```python
from build123d import *

# Parameters (mm, degrees)
SKETCH1_R           = 117.5
BOSS_EXTRUDE1_DEPTH = 5
SKETCH2_R           = 5.75
CUT_EXTRUDE1_DEPTH  = 167.245300685
CIRPATTERN1_COUNT   = 50
SKETCH3_R           = 6.25
CUT_EXTRUDE2_DEPTH  = 167.245300685
SKETCH4_R           = 2.25
CUT_EXTRUDE3_DEPTH  = 167.245300685
CIRPATTERN2_COUNT   = 4


with BuildPart() as part:
    # Sketch1 → Boss-Extrude1 (new body)
    with BuildSketch(Plane(origin=(0, 0, 0), x_dir=(1, 0, 0), z_dir=(0, 1, 0))):
        with Locations(Location((0, 0, 0), (0, 0, 270))):
            Circle(SKETCH1_R)
    extrude(amount=BOSS_EXTRUDE1_DEPTH)

    # Sketch2 → Cut-Extrude1 (cut, through all)
    with BuildSketch(Plane(origin=(0, 5, 0), x_dir=(1, 0, 0), z_dir=(0, 1, 0))):
        with Locations(Location((0, 107.5, 0), (0, 0, 270))):
            Circle(SKETCH2_R)
    cut_extrude1 = extrude(amount=-CUT_EXTRUDE1_DEPTH, mode=Mode.SUBTRACT)

    # CirPattern1: Cut-Extrude1 ×50 about axis
    cirpattern1_axis = Axis((0, 0, 0.258053464), (0, 1, 0))
    for i in range(1, CIRPATTERN1_COUNT):
        add(cut_extrude1.rotate(cirpattern1_axis, i * 360 / CIRPATTERN1_COUNT), mode=Mode.SUBTRACT)

    # Sketch3 → Cut-Extrude2 (cut, through all)
    with BuildSketch(Plane(origin=(0, 5, 0), x_dir=(1, 0, 0), z_dir=(0, 1, 0))):
        with Locations(Location((0, 0, 0), (0, 0, 270))):
            Circle(SKETCH3_R)
    extrude(amount=-CUT_EXTRUDE2_DEPTH, mode=Mode.SUBTRACT)

    # Sketch4 → Cut-Extrude3 (cut, through all)
    with BuildSketch(Plane(origin=(0, 5, 0), x_dir=(1, 0, 0), z_dir=(0, 1, 0))):
        with Locations(Location((19, 0, 0), (0, 0, 270))):
            Circle(SKETCH4_R)
    cut_extrude3 = extrude(amount=-CUT_EXTRUDE3_DEPTH, mode=Mode.SUBTRACT)

    # CirPattern2: Cut-Extrude3 ×4 about axis
    cirpattern2_axis = Axis((0, 0, 0), (0, 1, 0))
    for i in range(1, CIRPATTERN2_COUNT):
        add(cut_extrude3.rotate(cirpattern2_axis, i * 360 / CIRPATTERN2_COUNT), mode=Mode.SUBTRACT)


solid = part.part
```
Geometry check sheet. Reference: the model listing, model coordinates, mm. Coordinates: 2 decimals unless noted, no trailing zeros. Write each loop counter-clockwise with the first axis right and the second up, starting at its lowest first coordinate (ties: lowest second). Pieces come first, ordered by that corner, then holes. Notation, with made-up numbers: M 49,60 L 73,60 A10 cw 73,66 Z; hole C -8.75,-29 d2. An arc over 180 degrees is marked long. Answer as a JSON object with one key per item and string values.
1. Section check A-A, the plane z = -59.5. Enter the section's corners in (x, y), plus the area to 3 significant figures.
Answers below:
{"outline": "M -101.32,0 L -96.37,0 L -96.37,5 L -101.32,5 Z; M -85.6,0 L 85.6,0 L 85.6,5 L -85.6,5 Z; M 96.37,0 L 101.32,0 L 101.32,5 L 96.37,5 Z", "area": "906 mm²"}
2. Scan lines: L1, parallel to Z at x = 43, y = 1.45; L2, parallel to X at y = 0.6, z = 62; L3, parallel to Z at x = 63.5, y = 2.6. Record each from-to range of solid material in increasing order.
Answers below:
{"L1": "z = -109.35 to -104.62, -95.25 to 95.76, 105.14 to 109.35", "L2": "x = -99.81 to -95.11, -86.85 to 86.85, 95.11 to 99.81", "L3": "z = -98.86 to -92.67, -81.17 to 81.69, 93.18 to 98.86"}
3. Section check C-C, the plane y = 2.25. Give the number of separate pieces and of enclosed holes in the cut face, plus the area to 3 significant figures.
Answers below:
{"separate pieces": "1", "enclosed holes": "55", "area": "38,000 mm²"}
4. Draft check along X on faces 1 (the cylindrical face through (116.5, 2.5, -15.3)), 2 (the cylindrical face through (85.32, 2.54, -56.49)). Enter one of: released by +X, released by -X, zero draft, split by the parting line, or undercut.
Answers below:
{"face 1": "split by the parting line", "face 2": "undercut"}
5. Go/stop test with flat-tipped pins: pin 1 Ø18.5 at (x, z) = (-105.85, 20.45) entering from +Y; pin 2 Ø3 at (y, z) = (3, -87.5) entering from +X; pin 3 Ø3 at (y, z) = (0.5, -78.5) entering from +X. Record where each tip stops, or that it passes through.
Answers below:
{"pin 1": "stops at y = 5", "pin 2": "stops at x = 80.06", "pin 3": "stops at x = 88.75"}
6. Section check B-B, the plane z = 58. Enter the section's corners in (x, y).
Answers below:
{"outline": "M -102.19,0 L -96.73,0 L -96.73,5 L -102.19,5 Z; M -85.23,0 L 85.23,0 L 85.23,5 L -85.23,5 Z; M 96.73,0 L 102.19,0 L 102.19,5 L 96.73,5 Z"}
